Geometry check sheet. Reference: the model listing, model coordinates, mm. A direction names the side the tool comes from. Coordinates: 2 decimals unless noted, no trailing zeros. Write each loop counter-clockwise with the first axis right and the second up, starting at its lowest first coordinate (ties: lowest second). Pieces come first, ordered by that corner, then holes. Notation, with made-up numbers: (15, 88.25) -> (57, 88.25) arc R15 cw to (57, 101.25) -> close; hole circle Ø4 at (27.25, 62). An arc over 180 degrees is marked (long way). Use a Markdown table: item, result.
```python
from build123d import *

# Parameters (mm, degrees)
SKETCH1_W           = 25
SKETCH1_H           = 22
BOSS_EXTRUDE1_DEPTH = 60
CUT_EXTRUDE2_REACH  = 123.15
CUT_EXTRUDE3_REACH  = 123.15
SKETCH6_R           = 6.26
FILLET1_R           = 5
SKETCH2_R           = 3
BOSS_EXTRUDE2_DEPTH = 10
LPATTERN1_COUNT     = 6
LPATTERN1_PITCH     = 20
SKETCH3_R           = 3
BOSS_EXTRUDE3_DEPTH = 10
LPATTERN2_COUNT     = 6
LPATTERN2_PITCH     = 20
SKETCH9_R           = 7
SKETCH9_W           = 3
SKETCH9_H           = 11
CUT_EXTRUDE5_DEPTH  = 15


with BuildPart() as part:
    # Sketch1 → Boss-Extrude1 (new, symmetric)
    with BuildSketch(Plane(origin=(0, 0, 0), x_dir=(0, 0, -1), z_dir=(1, 0, 0))):
        Rectangle(SKETCH1_W, SKETCH1_H)
    extrude(amount=BOSS_EXTRUDE1_DEPTH, both=True)

    # Sketch5 → Cut-Extrude2 (cut, up to next)
    with BuildSketch(Plane(origin=(60, 0, 0), x_dir=(0, 0, -1), z_dir=(1, 0, 0)), mode=Mode.PRIVATE) as cut_extrude2_sk1:
        with BuildLine():
            Line((-13.743342576, 11), (-11.25, 11))
            Line((-11.25, 11), (-11.25, 6.005))
            ThreePointArc((-11.25, 6.005), (-23.092030441, 3.213639122), (-13.743342576, 11))
        make_face()
    cut_extrude2_tool1 = extrude(cut_extrude2_sk1.sketch, amount=-CUT_EXTRUDE2_REACH, mode=Mode.PRIVATE) & part.part
    add(cut_extrude2_tool1.solids().sort_by_distance((60, 6.117758, 17.335764))[0], mode=Mode.SUBTRACT)

    # Sketch6 → Cut-Extrude3 (cut, up to next)
    with BuildSketch(Plane.ZY.offset(60), mode=Mode.PRIVATE) as cut_extrude3_sk1:
        with Locations((18.339471377, -6)):
            Circle(SKETCH6_R)
    cut_extrude3_tool1 = extrude(cut_extrude3_sk1.sketch, amount=-CUT_EXTRUDE3_REACH, mode=Mode.PRIVATE) & part.part
    add(cut_extrude3_tool1.solids().sort_by_distance((-60, -6, 18.339471))[0], mode=Mode.SUBTRACT)

    # Fillet1
    fillet1_edges = [part.edges().sort_by_distance(p)[0] for p in [
        (0, 11, 11.25),
    ]]
    fillet(fillet1_edges, radius=FILLET1_R)

    # Sketch2 → Boss-Extrude2 (add)
    with BuildSketch(Plane(origin=(60, 0, 0), x_dir=(0, 0, -1), z_dir=(1, 0, 0))):
        with BuildLine():
            Line((-17.250000617, 1.202041029), (-6.000000617, 1.202041029))
            Line((-6.000000617, 1.202041029), (-6.000000617, 11))
            Line((-6.000000617, 11), (-17.250000617, 11))
            ThreePointArc((-17.250000617, 11), (-21.250000617, 6.101020514), (-17.250000617, 1.202041029))
        make_face()
        with Locations((-16.250000617, 6.101020514)):
            Circle(SKETCH2_R, mode=Mode.SUBTRACT)
    boss_extrude2 = extrude(amount=-BOSS_EXTRUDE2_DEPTH)

    # LPattern1: Boss-Extrude2 ×6
    with Locations(*[(-i * LPATTERN1_PITCH, 0, 0) for i in range(1, LPATTERN1_COUNT)]):
        add(boss_extrude2)

    # Sketch3 → Boss-Extrude3 (add)
    with BuildSketch(Plane.ZY.offset(60)):
        with BuildLine():
            Line((18.103250446, -1.202041029), (12.5, -1.202041029))
            Line((12.5, -1.202041029), (12.5, -3.744301875))
            ThreePointArc((12.5, -3.744301875), (12.185501487, -4.85271861), (12.079471377, -6))
            ThreePointArc((12.079471377, -6), (12.185501487, -7.14728139), (12.5, -8.255698125))
            Line((12.5, -8.255698125), (12.5, -11))
            Line((12.5, -11), (18.103250446, -11))
            ThreePointArc((18.103250446, -11), (22.103250446, -6.101020514), (18.103250446, -1.202041029))
        make_face()
        with Locations((17.103250446, -6.101020514)):
            Circle(SKETCH3_R, mode=Mode.SUBTRACT)
    boss_extrude3 = extrude(amount=-BOSS_EXTRUDE3_DEPTH)

    # LPattern2: Boss-Extrude3 ×6
    with Locations(*[(i * LPATTERN2_PITCH, 0, 0) for i in range(1, LPATTERN2_COUNT)]):
        add(boss_extrude3)

    # Sketch9 → Cut-Extrude5 (cut)
    with BuildSketch(Plane(origin=(0, 0, -12.5), x_dir=(-1, 0, 0), z_dir=(0, 0, -1))):
        with Locations(Location((0, 0, 0), (0, 0, 90))):
            Circle(SKETCH9_R)
        with Locations((-14, 0)):
            Rectangle(SKETCH9_W, SKETCH9_H)
        with Locations((14, 0)):
            Rectangle(SKETCH9_W, SKETCH9_H)
    extrude(amount=-CUT_EXTRUDE5_DEPTH, mode=Mode.SUBTRACT)


solid = part.part
```
Item 1: Depth check by flat-ended pin: P1, Ø1.4, axis at x = 52.5, z = 14, coming from the -Y side; P2, Ø4, axis at y = 7.5, z = 18.5, coming from the -X side; P3, Ø5, axis at y = -6.1, z = 17.1, coming from the +X side; P4, Ø3, axis at y = -3.5, z = 17.5, coming from the +X side. Enter the tip coordinate at first touch or a pass-through.
Answer block:
| item | result |
|---|---|
| P1 | stops at y = 1.2 |
| P2 | stops at x = -50 |
| P3 | passes through |
| P4 | stops at x = 50 |
Item 2: Mould release check, pull along X, two halves, no side actions. Record for faces 5 (the flat face through (5, -1.202, 15)), 6 (the flat face through (50, -3.9, 14.8)), 7 (the cylindrical face through (5.07, 4.054, 11.562)): +X half, -X half, draft (parallel to the pull), parting line (faces both ways), or undercut.
Answer block:
| item | result |
|---|---|
| face 5 | draft |
| face 6 | +X half |
| face 7 | undercut |
Item 3: Section check B-B on y = 0. Record the boundary of the cut face in (x, z), then the cut area to 3 significant figures.
Answer block:
| item | result |
|---|---|
| outline | (-60, -12.5) -> (-15.5, -12.5) -> (-15.5, 2.5) -> (-12.5, 2.5) -> (-12.5, -12.5) -> (-7, -12.5) -> (-7, 2.5) -> (7, 2.5) -> (7, -12.5) -> (12.5, -12.5) -> (12.5, 2.5) -> (15.5, 2.5) -> (15.5, -12.5) -> (60, -12.5) -> (60, 12.5) -> (-60, 12.5) -> close |
| area | 2,700 mm^2 |
Item 4: Tool access check on faces 1 (the flat face through (-15, -1.202, 15)), 2 (the flat face through (-15.5, 0, -5)), 3 (the flat face through (35, -10, 12.5)), 4 (the flat face through (10, 8.3, 13.9)). Record the directions out of +Z, -Z, +X, -X, +Y, -Y that give a thin tool (end or side, any length) a straight path to the whole face; none if there is none.
Answer block:
| item | result |
|---|---|
| face 1 | +Z, +X, -X, +Y |
| face 2 | -Z |
| face 3 | +Z, -Y |
| face 4 | +Z, +Y |
Item 5: Section check C-C on x = 14. Record the boundary of the cut face in (y, z), then the cut area to 3 significant figures.
Answer block:
| item | result |
|---|---|
| outline | (-11, -12.5) -> (-5.5, -12.5) -> (-5.5, 2.5) -> (5.5, 2.5) -> (5.5, -12.5) -> (11, -12.5) -> (11, 17.25) arc R5 ccw to (1.2, 17.25) -> (1.2, 12.5) -> (-3.74, 12.5) arc R6.26 cw to (-8.26, 12.5) -> (-11, 12.5) -> close; hole circle Ø6 at (6.1, 16.25) |
| area | 431 mm^2 |
Item 6: Section check A-A on x = -46. Record the boundary of the cut face in (y, z).
Answer block:
| item | result |
|---|---|
| outline | (-11, -12.5) -> (11, -12.5) -> (11, 17.25) arc R5 ccw to (1.2, 17.25) -> (1.2, 12.5) -> (-3.74, 12.5) arc R6.26 cw to (-8.26, 12.5) -> (-11, 12.5) -> close; hole circle Ø6 at (6.1, 16.25) |
Item 7: Thickness scan on L1, parallel to X at y = 7.75, z = 13; L2, parallel to X at y = -5.75, z = 21; L3, parallel to Y at x = 54, z = 16. Record the ranges inside material, lowest first. Write a range as [from, to].
Answer block:
| item | result |
|---|---|
| L1 | x = [-50, -40], [-30, -20], [-10, 0], [10, 20], [30, 40], [50, 60] |
| L2 | x = [-60, -50], [-40, -30], [-20, -10], [0, 10], [20, 30], [40, 50] |
| L3 | y = [1.2, 3.11], [9.09, 11] |
